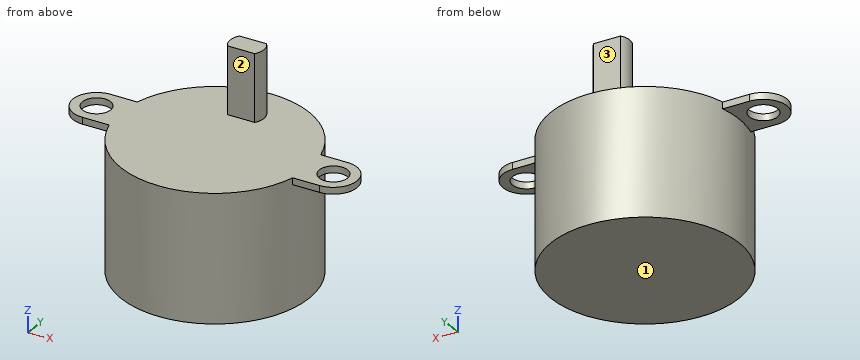
```python
from build123d import *

# Parameters (mm, degrees)
SKETCH_R     = 14
PAD_DEPTH    = 19
PAD001_DEPTH = 10
SKETCH002_R  = 2.1
PAD002_DEPTH = 1


with BuildPart() as part:
    # Sketch → Pad (new body)
    with BuildSketch(Plane.XY):
        Circle(SKETCH_R)
    extrude(amount=PAD_DEPTH)

    # Sketch001 → Pad001 (new body)
    with BuildSketch(Plane.XY.offset(19)):
        with BuildLine():
            ThreePointArc((-2, 9.5), (-2.5, 8), (-2, 6.5))
            Line((2, 6.5), (-2, 6.5))
            ThreePointArc((2, 6.5), (2.5, 8), (2, 9.5))
            Line((-2, 9.5), (2, 9.5))
        make_face()
    extrude(amount=PAD001_DEPTH)

    # Sketch002 → Pad002 (new body)
    with BuildSketch(Plane.XY.offset(19)):
        with BuildLine():
            ThreePointArc((-17.5, 3.5), (-21, 0), (-17.5, -3.5))
            Line((-17.5, -3.5), (17.5, -3.5))
            ThreePointArc((17.5, -3.5), (21, 0), (17.5, 3.5))
            Line((-17.5, 3.5), (17.5, 3.5))
        make_face()
        with Locations((-17.5, 0)):
            Circle(SKETCH002_R, mode=Mode.SUBTRACT)
        with Locations((17.5, 0)):
            Circle(SKETCH002_R, mode=Mode.SUBTRACT)
    extrude(amount=-PAD002_DEPTH)


solid = part.part
```
Design review of the part built by this model. Coordinates are the model's own, in mm. Face numbers are marked on the shaded views. A direction names the side the tool comes from. Give positions to 0.01 mm unless a question says otherwise; leave off trailing zeros. Order: outer loops, then holes, each group sorted by start corner. A loop starts at its lowest first (then second) coordinate and runs counter-clockwise, first axis right, second up. Notation, with made-up numbers: (-1.75, 15.25) -> (28.25, 15.25) arc R25 ccw to (28.25, 43.25) -> close; hole circle Ø7 at (12, 41). An arc over 180 degrees is marked (long way). Write each question's results on one line, items separated by ' | '. Start each with the question number.
Q1. Add section B-B on x = 17. Give the boundary of the cut face in (y, z), and give its area (3 significant figures).
Q2. Add section C-C on z = 27.25. Give the boundary of the cut face in (x, y).
Q3. Add section A-A on y = 0. Give the boundary of the cut face in (x, z), and give its area (3 significant figures).
Q4. For pin 1 (8 mm diameter, centred on y = -4, z = 17.5, fed in from +X); pin 2 (7.5 mm diameter, centred on x = 18.5, y = 1.5, fed in from -Z); pin 3 (6 mm diameter, centred on x = -4, z = 24, fed in from +Y); pin 4 (1.1 mm diameter, centred on x = -16, z = 18.5, fed in from +Y), all flat-tipped, find the tip position at first contact; note any pin that passes through.
Q5. Wall thickness on L1, parallel to Y at x = 17.5, z = 18.2; L2, parallel to Y at x = -0.5, z = 26.25; L3, parallel to X at y = 8, z = 21.25: over which ranges is each line inside the solid? List them lowest first. Write a range as from..to.
Q6. Add section D-D on x = 0. Give the boundary of the cut face in (y, z).
Q7. Machinability: for the marked faces 1, 2 and 3, which of the approach directions +Z, -Z, +X, -X, +Y, -Y give a long, thin tool a straight path to every point of the face, cutting with its end or side? Answer none if there is none.
Found:
1) outline: (-3.5, 18) -> (-2.04, 18) -> (-2.04, 19) -> (-3.5, 19) -> close; (2.04, 18) -> (3.5, 18) -> (3.5, 19) -> (2.04, 19) -> close | area: 2.92 mm2
2) outline: (-2, 6.5) -> (2, 6.5) arc R2.5 ccw to (2, 9.5) -> (-2, 9.5) arc R2.5 ccw to start
3) outline: (-21, 18) -> (-19.6, 18) -> (-19.6, 19) -> (-21, 19) -> close; (-15.4, 18) -> (-14, 18) -> (-14, 0) -> (14, 0) -> (14, 18) -> (15.4, 18) -> (15.4, 19) -> (-15.4, 19) -> close; (19.6, 18) -> (21, 18) -> (21, 19) -> (19.6, 19) -> close | area: 538 mm2
4) pin 1: stops at x = 21 | pin 2: stops at z = 18 | pin 3: stops at y = 9.5 | pin 4: stops at y = 3.5
5) L1: y = -3.5..-2.1, 2.1..3.5 | L2: y = 6.5..9.5 | L3: x = -2.5..2.5
6) outline: (-14, 0) -> (14, 0) -> (14, 19) -> (9.5, 19) -> (9.5, 29) -> (6.5, 29) -> (6.5, 19) -> (-14, 19) -> close
7) face 1: -Z, +X, -X, +Y, -Y | face 2: +Z, +X, -X, -Y | face 3: +Z, +X, -X, +Y
